Input: part model. Units: mm. Frame: model coordinates. A direction names the side the tool comes from. Round coordinates to 2 decimals unless told otherwise and drop trailing zeros. Order: outer loops, then holes, each group sorted by start corner. A loop starts at its lowest first (then second) coordinate and runs counter-clockwise, first axis right, second up. Notation, with made-up numbers: (83.5, 37.25) -> (141.5, 37.25) arc R19 ccw to (141.5, 66.25) -> close; hole circle Ø11 at (-20, 21.5). An arc over 180 degrees is marked (long way). Answer as CSV lines item,"result". Start each with the question number.
1) Section query A-A, the plane x = 4. Output: boundary loops of the cut face in (y, z), and give its area (3 significant figures).
2) Line query: L1, parallel to X at y = -14, z = 46.5; L2, parallel to Y at x = 16, z = 37; L3, parallel to Y at x = 48, z = 20. Output: solid intervals per line, ascending.
3) First-contact query: P1, Ø4, axis at x = 36.5, z = 13.5, coming from the -Y side; P2, Ø1.5, axis at y = -10.5, z = 40.5, coming from the +X side. Flat tips, straight axial feed; report the tip coordinate or a pass-through.
4) Mould query, pull axis X, two halves, no side actions, for faces 3 (the face through (48, -1, 25)), 4 (the face through (46, -16.5, 4)), 5 (the face through (3.759, -12.958, 5.834)). Classes: +X half, -X half, draft (parallel to the pull), parting line (faces both ways), or undercut.
5) Access query for faces 1 (the face through (49, -6, 2)), 2 (the face through (44.15, -12.96, 4.08)). Directions: +Z, -Z, +X, -X, +Y, -Y. A direction counts if a zero-diameter tool reaches every point of the face in a straight line with its end or side. Return the directions, or none.
6) Section query D-D, the plane z = 33. Output: boundary loops of the cut face in (x, y).
7) Section query B-B, the plane z = 46. Output: boundary loops of the cut face in (x, y).
8) Section query C-C, the plane y = -14.5. Output: boundary loops of the cut face in (x, z), and give its area (3 significant figures).
```python
from build123d import *

# Parameters (mm, degrees)
F0_W     = 50
F0_H     = 50
F1_DEPTH = 10
F2_R     = 1.85
F3_DEPTH = 6.5
F4_SIZE  = 0.5
F5_SIZE  = 3


with BuildPart() as f1:
    # F0 (on Front) → F1 (new body)
    with BuildSketch(Plane.XZ):
        with Locations((25, 25)):
            Rectangle(F0_W, F0_H)
    extrude(amount=F1_DEPTH)

    # F2 (on face) → F3 (join)
    with BuildSketch(Plane.XZ.offset(10)):
        with Locations((4, 46)):
            Circle(F2_R)
        with Locations((46, 46)):
            Circle(F2_R)
        with Locations((46, 4)):
            Circle(F2_R)
        with Locations((4, 4)):
            Circle(F2_R)
    extrude(amount=F3_DEPTH)

    # F4
    f4_edges = [f1.edges().sort_by_distance(p)[0] for p in [
        (2.15, -16.5, 4),
        (44.15, -16.5, 4),
        (44.15, -16.5, 46),
        (2.15, -16.5, 46),
    ]]
    chamfer(f4_edges, length=F4_SIZE)

    # F5
    f5_edges = [f1.edges().sort_by_distance(p)[0] for p in [
        (0, -5, 50),
        (50, -5, 50),
        (50, -5, 0),
        (0, -5, 0),
        (0, 0, 25),
        (25, 0, 0),
        (50, 0, 25),
        (25, 0, 50),
    ]]
    chamfer(f5_edges, length=F5_SIZE)


solid = f1.part
```
Findings:
1,outline,"(-16.5, 2.65) -> (-16, 2.15) -> (-10, 2.15) -> (-10, 0) -> (-3, 0) -> (0, 3) -> (0, 47) -> (-3, 50) -> (-10, 50) -> (-10, 47.85) -> (-16, 47.85) -> (-16.5, 47.35) -> (-16.5, 44.65) -> (-16, 44.15) -> (-10, 44.15) -> (-10, 5.85) -> (-16, 5.85) -> (-16.5, 5.35) -> close"
1,area,"539 mm^2"
2,L1,"x = 2.22 to 5.78, 44.22 to 47.78"
2,L2,"y = -10 to 0"
2,L3,"y = -10 to -1"
3,P1,"stops at y = -10"
3,P2,"stops at x = 50"
4,face 3,"+X half"
4,face 4,"draft"
4,face 5,"undercut"
5,face 1,"-Z, +X, +Y, -Y"
5,face 2,"-Y"
6,outline,"(0, -10) -> (50, -10) -> (50, -3) -> (47, 0) -> (3, 0) -> (0, -3) -> close"
7,outline,"(0, -10) -> (2.15, -10) -> (2.15, -16) -> (2.65, -16.5) -> (5.35, -16.5) -> (5.85, -16) -> (5.85, -10) -> (44.15, -10) -> (44.15, -16) -> (44.65, -16.5) -> (47.35, -16.5) -> (47.85, -16) -> (47.85, -10) -> (50, -10) -> (50, -3) -> (47, 0) -> (3, 0) -> (0, -3) -> close"
8,outline,"circle Ø3.7 at (4, 4); circle Ø3.7 at (4, 46); circle Ø3.7 at (46, 4); circle Ø3.7 at (46, 46)"
8,area,"43.0 mm^2"
